Geometry: final body of the model. Coordinates: model frame, mm. A direction names the side the tool comes from. Give positions to 0.01 mm unless a question says otherwise; leave off trailing zeros. Write each loop counter-clockwise with the first axis right and the second up, starting at its lowest first coordinate (ties: lowest second). Pieces come first, ordered by that corner, then holes. Notation, with made-up numbers: (-8.75, -1.5) -> (42.25, -1.5) arc R8 ccw to (42.25, 2.5) -> close; hole circle Ø6 at (64, -16). An arc over 180 degrees is marked (long way). Use CSV: the item, a comma, the result in double quotes. Start each with the question number.
1) Section C-C (x = -71). Output: boundary loops of the cut face in (y, z).
2) Set-up query: faces 5 (the face through (-67.55, 64, 2)), 6 (the face through (-16.55, 52, 2)), 7 (the face through (-12.8, 82.4, 7)), 8 (the face through (-16.327, 21.43, 5.986)). Return all of +Z, -Z, +X, -X, +Y, -Y with unobstructed straight access to the full face (end or side cutting, diameter ignored); none if empty.
3) Section A-A (x = -39). Output: boundary loops of the cut face in (y, z), plus the area to 3 significant figures.
4) Section B-B (y = 64.5). Output: boundary loops of the cut face in (x, z).
5) Draft query along X for faces 1 (the face through (-59.55, 52, 2)), 2 (the face through (34.696, -11.494, 2.465)), 3 (the face through (52.08, 8.45, 2.46)), 4 (the face through (-85.5, 31.5, 2.5)). Return one class per face: pulls with the +X half, pulls with the -X half, needs draft (parallel to the pull), parting line crosses it, or undercut.
6) Contact query for flat-ended pins moving along their axis: P1, Ø4, axis at x = -27.5, z = 2, coming from the -Y side; P2, Ø1, axis at x = 21, y = 69, coming from the +Z side; P3, Ø1, axis at y = 11.5, z = 3, coming from the +X side. Output: stop coordinate, or through.
7) Material intervals for line 1 (Y direction, x = -62.55, z = 2.5); line 2 (Z direction, x = 42.75, y = -4); line 3 (X direction, y = 64, z = 1.5), sorted ascending. Write a range as [from, to].
```python
from build123d import *

# Parameters (mm, degrees)
SKETCH1_R               = 0.95
SKETCH1_W               = 6.5
SKETCH1_H               = 6.5
SKETCH1_R_2             = 1.55
SKETCH1_R_3             = 1.45
SKETCH1_W_2             = 43
SKETCH1_H_2             = 52
BOSS_EXTRUDE1_DEPTH     = 5
SKETCH3_R               = 5
SKETCH3_R_2             = 1.45
SKETCH3_R_3             = 5.5
SKETCH3_R_4             = 3.5
SKETCH3_R_5             = 0.95
BOSS_EXTRUDE3_DEPTH     = 2
CUT_EXTRUDE1_DEPTH      = 10
SKETCH6_R               = 1
CUT_EXTRUDE2_DEPTH      = 14.13
CUT_EXTRUDE2_DEPTH_BACK = 10


with BuildPart() as part:
    # Sketch1 → Boss-Extrude1 (new body)
    with BuildSketch(Plane.XY):
        with BuildLine():
            Line((13.24210093, 18.56), (28.512575376, -7.763418891))
            ThreePointArc((28.512575376, -7.763418891), (34.802937336, -11.49741064), (41.280767541, -8.099019285))
            Line((41.280767541, -8.099019285), (63.187178361, 25.467320477))
            ThreePointArc((63.187178361, 25.467320477), (63.966953059, 27.626085973), (63.700028418, 29.905793912))
            Line((63.700028418, 29.905793912), (42.050042627, 89.558690868))
            ThreePointArc((42.050042627, 89.558690868), (36.572238317, 94.333353031), (29.618521803, 92.223953715))
            Line((29.618521803, 92.223953715), (24.120361081, 86.56))
            Line((24.120361081, 86.56), (-63.55, 86.56))
            ThreePointArc((-63.55, 86.56), (-66.378427125, 85.388427125), (-67.55, 82.56))
            Line((-67.55, 82.56), (-67.55, 44.56))
            Line((-67.55, 44.56), (-92.289702732, 34.753715855))
            ThreePointArc((-92.289702732, 34.753715855), (-94.499992282, 31.492649998), (-92.276025776, 28.240896102))
            Line((-92.276025776, 28.240896102), (-67.55, 18.56))
            Line((-67.55, 18.56), (13.24210093, 18.56))
        make_face()
        with Locations((-62.55, 23.56)):
            Circle(SKETCH1_R, mode=Mode.SUBTRACT)
        with BuildLine():
            ThreePointArc((-87, 32.997152184), (-85.5, 31.497152184), (-87, 29.997152184))
            Line((-87, 29.997152184), (-91, 29.997152184))
            Line((-91, 29.997152184), (-91, 30))
            ThreePointArc((-91, 30), (-92.5, 31.5), (-91, 33))
            Line((-91, 33), (-87, 33))
            Line((-87, 33), (-87, 32.997152184))
        make_face(mode=Mode.SUBTRACT)
        with BuildLine():
            Line((-67.55, 23.929574136), (-83.648509217, 30.232568258))
            ThreePointArc((-83.648509217, 30.232568258), (-83.407620833, 31.515944037), (-83.65389726, 32.798296766))
            Line((-83.65389726, 32.798296766), (-67.55, 39.18153403))
            Line((-67.55, 39.18153403), (-67.55, 23.929574136))
        make_face(mode=Mode.SUBTRACT)
        with Locations((35, -4)):
            Rectangle(SKETCH1_W, SKETCH1_H, mode=Mode.SUBTRACT)
        with Locations((11, 29.4)):
            Circle(SKETCH1_R_2, mode=Mode.SUBTRACT)
        with Locations((59, 28.2)):
            Circle(SKETCH1_R_3, mode=Mode.SUBTRACT)
        with Locations((-38.05, 52.56)):
            Rectangle(SKETCH1_W_2, SKETCH1_H_2, mode=Mode.SUBTRACT)
        with Locations((-62.55, 81.56)):
            Circle(SKETCH1_R, mode=Mode.SUBTRACT)
        with BuildLine():
            ThreePointArc((7.606653519, 30.257437846), (7.500011538, 29.408987159), (7.602294892, 28.56))
            Line((7.602294892, 28.56), (-9.55, 28.56))
            Line((-9.55, 28.56), (-9.55, 80.56))
            Line((-9.55, 80.56), (20.317209538, 80.56))
            Line((20.317209538, 80.56), (7.606653519, 30.257437846))
        make_face(mode=Mode.SUBTRACT)
        with Locations((-13.55, 81.56)):
            Circle(SKETCH1_R, mode=Mode.SUBTRACT)
        with Locations((26, 80.6)):
            Circle(SKETCH1_R_3, mode=Mode.SUBTRACT)
        with Locations((35, 87)):
            Rectangle(SKETCH1_W, SKETCH1_H, mode=Mode.SUBTRACT)
        with Locations((-13.55, 23.56)):
            Circle(SKETCH1_R, mode=Mode.SUBTRACT)
    extrude(amount=BOSS_EXTRUDE1_DEPTH)

    # Sketch3 → Boss-Extrude3 (add)
    with BuildSketch(Plane.XY.offset(5)):
        with Locations((59, 28.2)):
            Circle(SKETCH3_R)
        with Locations((59, 28.2)):
            Circle(SKETCH3_R_2, mode=Mode.SUBTRACT)
        with Locations((26, 80.6)):
            Circle(SKETCH3_R_3)
        with Locations((26, 80.6)):
            Circle(SKETCH3_R_2, mode=Mode.SUBTRACT)
        with BuildLine():
            ThreePointArc((12.55, 29.4), (10.347121757, 27.994208408), (10, 30.584271928))
            Line((10, 30.584271928), (10, 32.754101966))
            ThreePointArc((10, 32.754101966), (8.473400258, 31.822043299), (7.606653519, 30.257437846))
            ThreePointArc((7.606653519, 30.257437846), (7.500011538, 29.408987159), (7.602294892, 28.56))
            ThreePointArc((7.602294892, 28.56), (13.415547613, 26.867189362), (12, 32.754101966))
            Line((12, 32.754101966), (12, 30.584271928))
            ThreePointArc((12, 30.584271928), (12.405791592, 30.052878243), (12.55, 29.4))
        make_face()
        with Locations((-13.55, 23.56)):
            Circle(SKETCH3_R_4)
        with Locations((-13.55, 23.56)):
            Circle(SKETCH3_R_5, mode=Mode.SUBTRACT)
        with Locations((-62.55, 23.56)):
            Circle(SKETCH3_R_4)
        with Locations((-62.55, 23.56)):
            Circle(SKETCH3_R_5, mode=Mode.SUBTRACT)
        with Locations((-62.55, 81.56)):
            Circle(SKETCH3_R_4)
        with Locations((-62.55, 81.56)):
            Circle(SKETCH3_R_5, mode=Mode.SUBTRACT)
        with Locations((-13.55, 81.56)):
            Circle(SKETCH3_R_4)
        with Locations((-13.55, 81.56)):
            Circle(SKETCH3_R_5, mode=Mode.SUBTRACT)
    extrude(amount=BOSS_EXTRUDE3_DEPTH)

    # Sketch4 → Cut-Extrude1 (cut)
    with BuildSketch(Plane.XY.offset(5)):
        Polygon((34.174437675, 81.42265859), (52.588350326, 30.686217258), (34.375314724, 2.779092439), (20.392987639, 26.881988144), align=None)
    extrude(amount=-CUT_EXTRUDE1_DEPTH, mode=Mode.SUBTRACT)

    # Sketch6 → Cut-Extrude2 (cut, two sides)
    with BuildSketch(Plane.ZY.offset(-38.25)) as cut_extrude2_sk:
        with Locations((2.5, -4)):
            Circle(SKETCH6_R)
        with Locations((2.5, 87)):
            Circle(SKETCH6_R)
    extrude(amount=CUT_EXTRUDE2_DEPTH, mode=Mode.SUBTRACT)
    extrude(cut_extrude2_sk.sketch, amount=-CUT_EXTRUDE2_DEPTH_BACK, mode=Mode.SUBTRACT)


solid = part.part
```
Answers follow:
1,outline,"(19.91, 0) -> (25.28, 0) -> (25.28, 5) -> (19.91, 5) -> close; (37.81, 0) -> (43.19, 0) -> (43.19, 5) -> (37.81, 5) -> close"
2,face 5,"+Z, -Z, -X, +Y"
2,face 6,"+Z, -Z"
2,face 7,"+Z, +X, -X, +Y, -Y"
2,face 8,"+Z"
3,outline,"(18.56, 0) -> (26.56, 0) -> (26.56, 5) -> (18.56, 5) -> close; (78.56, 0) -> (86.56, 0) -> (86.56, 5) -> (78.56, 5) -> close"
3,area,"80.0 mm^2"
4,outline,"(-67.55, 0) -> (-59.55, 0) -> (-59.55, 5) -> (-67.55, 5) -> close; (-16.55, 0) -> (-9.55, 0) -> (-9.55, 5) -> (-16.55, 5) -> close; (16.26, 0) -> (29.9, 0) -> (29.9, 5) -> (16.26, 5) -> close; (40.32, 0) -> (51.14, 0) -> (51.14, 5) -> (40.32, 5) -> close"
5,face 1,"undercut"
5,face 2,"parting line crosses it"
5,face 3,"pulls with the +X half"
5,face 4,"undercut"
6,P1,"stops at y = 18.56"
6,P2,"stops at z = 5"
6,P3,"stops at x = 54.4"
7,line 1,"y = [18.56, 22.61], [24.51, 80.61], [82.51, 86.56]"
7,line 2,"z = [0, 1.5], [3.5, 5]"
7,line 3,"x = [-67.55, -59.55], [-16.55, -9.55], [16.13, 29.77], [40.5, 51.33]"
